Can you work these out from the model? Positions are in its coordinate system, mm. Coordinates: 2 decimals unless noted, no trailing zeros. Loops run counter-clockwise (first coordinate to the right, second up) from the corner with the lowest first, then second, coordinate; pieces in that order, holes last. Notation, with made-up numbers: M -15,-3.5 L 18,-3.5 A24 ccw 18,18.5 Z; hole C 15.5,21.25 d3. An arc over 180 degrees is marked long. Return JSON: item names as keys, results as strings. Group by question number.
```python
from build123d import *

# Parameters (mm, degrees)
F0_R     = 1.5
F1_DEPTH = 1.2


with BuildPart() as f1:
    # F0 (on Top) → F1 (new body)
    with BuildSketch(Plane.XY):
        with BuildLine():
            Line((-9.5, 0), (9.5, 0))
            ThreePointArc((9.5, 0), (0, 9.5), (-9.5, 0))
        make_face()
        with BuildLine():
            ThreePointArc((-9.5, 0), (0, -9.5), (9.5, 0))
            Line((9.5, 0), (-9.5, 0))
        make_face()
        with BuildLine():
            Line((9.5, -13), (9.5, 0))
            ThreePointArc((9.5, 0), (0, -9.5), (-9.5, 0))
            Line((-9.5, 0), (-9.5, -13))
            Line((-9.5, -13), (9.5, -13))
        make_face()
        with Locations((-6.5, -10)):
            Circle(F0_R, mode=Mode.SUBTRACT)
        with Locations((6.5, -10)):
            Circle(F0_R, mode=Mode.SUBTRACT)
    extrude(amount=F1_DEPTH)


solid = f1.part
```
1) If we mould it in two halves opening along Y, with no side actions, what happens to faces 1 (the face through (0.209, 9.498, 0.592)), 2 (the face through (0, -2, 1.2)), 3 (the face through (-7.7, -10.9, 0.6))? For each: +Y half, -Y half, draft (parallel to the pull), parting line (faces both ways), or undercut.
2) Suppose I cut it at D-D, the plane y = 6.5. List the corners of the cut face in (x, z) for me.
3) Suppose I cut it at A-A, the plane z = 0.7. List the corners of the cut face in (x, y) for me.
4) Suppose I cut it at B-B, the plane x = -6.5. List the corners of the cut face in (y, z) for me.
5) If I drill on line 1 (Y direction, x = -6.5, z = 0.4); line 2 (Y direction, x = 1, z = 0.75); line 3 (X direction, y = 0.5, z = 1.1), over which ranges is the centre line in solid material (lowest first)? Write a range as from..to.
6) Suppose I cut it at C-C, the plane x = 7.5. List the corners of the cut face in (y, z) for me.
Returned:
{
 "1": {"face 1": "+Y half", "face 2": "draft", "face 3": "undercut"},
 "2": {"outline": "M -6.93,0 L 6.93,0 L 6.93,1.2 L -6.93,1.2 Z"},
 "3": {"outline": "M -9.5,-13 L 9.5,-13 L 9.5,0 A9.5 ccw -9.5,0 Z; hole C -6.5,-10 d3; hole C 6.5,-10 d3"},
 "4": {"outline": "M -13,0 L -11.5,0 L -11.5,1.2 L -13,1.2 Z; M -8.5,0 L 6.93,0 L 6.93,1.2 L -8.5,1.2 Z"},
 "5": {"line 1": "y = -13..-11.5, -8.5..6.93", "line 2": "y = -13..9.45", "line 3": "x = -9.49..9.49"},
 "6": {"outline": "M -13,0 L -11.12,0 L -11.12,1.2 L -13,1.2 Z; M -8.88,0 L 5.83,0 L 5.83,1.2 L -8.88,1.2 Z"}
}
